Verification items for the finished model (mm, model axes). Face numbers are marked on the shaded views. Give positions to 0.01 mm unless a question says otherwise; leave off trailing zeros. Loops run counter-clockwise (first coordinate to the right, second up) from the corner with the lowest first, then second, coordinate; pieces in that order, holes last. Notation, with made-up numbers: (74.5, 47.25) - (133.5, 47.25) arc R11 cw to (133.5, 65.25) - close; hole circle Ø7 at (81, 78). An arc over 180 degrees is marked (long way). Answer in a Markdown table with one row per item.
```python
from build123d import *

# Parameters (mm, degrees)
F0_R     = 40.1475524572
F0_R_2   = 26.11755
F1_DEPTH = 1.524
F2_DEPTH = 6.096


# Not quite as in the source:
# - a fillet or chamfer that OpenCascade refuses, or shapes differently, is made with other operations: its cross-section is extruded or revolved along the edge and cut away or added


with BuildPart() as f1:
    # F0 (on Front) → F1 (new body)
    with BuildSketch(Plane.XZ):
        Circle(F0_R)
        with Locations((0.0001517863, 0)):
            Circle(F0_R_2, mode=Mode.SUBTRACT)
        with Locations((0.0001517863, 0)):
            Circle(F0_R_2)
        with BuildLine():
            ThreePointArc((0.0001517863, 22.3475835458), (14.93341969, 16.1620214495), (21.1189817863, 1.2287535458))
            ThreePointArc((21.1189817863, 1.2287535458), (-14.9331161175, -13.704514358), (0.0001517863, 22.3475835458))
        make_face(mode=Mode.SUBTRACT)
    extrude(amount=F1_DEPTH)

    # F0 (on Front) → F2 (join)
    with BuildSketch(Plane.XZ):
        with Locations((0.0001517863, 0)):
            Circle(F0_R_2)
        with BuildLine():
            ThreePointArc((0.0001517863, 22.3475835458), (14.93341969, 16.1620214495), (21.1189817863, 1.2287535458))
            ThreePointArc((21.1189817863, 1.2287535458), (-14.9331161175, -13.704514358), (0.0001517863, 22.3475835458))
        make_face(mode=Mode.SUBTRACT)
    extrude(amount=F2_DEPTH)

    # F3: fillet of radius 5.08 on 1 edges, made by hand

    # F3_s1 → F3_t2 (revolve)
    with BuildSketch(Plane.XY):
        with BuildLine():
            ThreePointArc((31.1722379668, -1.524), (27.764470369, -2.8365711686), (26.1177017863, -6.096))
            Line((26.1177017863, -6.096), (26.1177017863, -1.524))
            Line((26.1177017863, -1.524), (31.1722379668, -1.524))
        make_face()
    revolve(axis=Axis((0.0001517863, -1.524, 0), (0, 1, 0)))


solid = f1.part
```
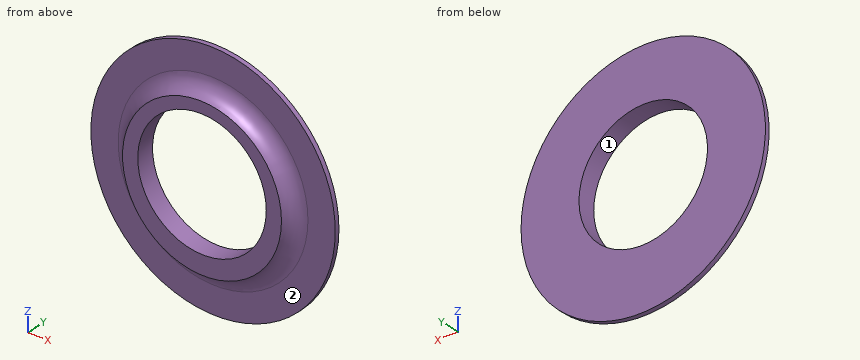
Q1. Go/stop test with flat-tipped pins: P1, Ø3, axis at x = 9.5, z = 26.5, coming from the -Y side; P2, Ø1.5, axis at x = 15, y = -4.5, coming from the -Z side; P3, Ø24, axis at x = 19.5, z = -6, coming from the -Y side; P4, Ø1, axis at x = -27.5, y = -1, coming from the +Z side. Record where each tip stops, or that it passes through.
Completed:
| item | result |
|---|---|
| P1 | y = -4.29 |
| P2 | z = -22.59 |
| P3 | y = -6.1 |
| P4 | z = 29.71 |
Q2. Sectioned sample at C-C (y = -4). Record the cut outline in (x, z).
Completed:
| item | result |
|---|---|
| outline | circle Ø53.62 at (0, 0); hole circle Ø42.24 at (0, 1.23) |
Q3. Sectioned sample at B-B (x = -34). Record the cut outline in (y, z).
Completed:
| item | result |
|---|---|
| outline | (-1.52, -21.35) - (0, -21.35) - (0, 21.35) - (-1.52, 21.35) - close |
Q4. Draft check along X on the marked faces 1 and 2. Enter one of: +X half, -X half, draft (parallel to the pull), parting line (faces both ways), or undercut.
Completed:
| item | result |
|---|---|
| face 1 | undercut |
| face 2 | draft |
Q5. Sectioned sample at D-D (z = 33). Record the cut outline in (x, y), and give its area (3 significant figures).
Completed:
| item | result |
|---|---|
| outline | (-22.87, -1.52) - (22.87, -1.52) - (22.87, 0) - (-22.87, 0) - close |
| area | 69.7 mm^2 |
Q6. Thickness scan on line 1 (X direction, y = -1.25, z = -30.5); line 2 (Z direction, x = -10.5, y = -2.5); line 3 (Z direction, x = -6.5, y = -5.5). Record the ranges inside material, lowest first.
Completed:
| item | result |
|---|---|
| line 1 | -26.11 to 26.11 |
| line 2 | -26.15 to -17.09, 19.55 to 26.15 |
| line 3 | -25.39 to -18.86, 21.32 to 25.39 |
Q7. Sectioned sample at A-A (z = 0). Record the cut outline in (x, y), and give its area (3 significant figures).
Completed:
| item | result |
|---|---|
| outline | (-40.15, -1.52) - (-31.17, -1.52) arc R5.08 cw to (-26.12, -6.1) - (-21.08, -6.1) - (-21.08, 0) - (-40.15, 0) - close; (21.08, -6.1) - (26.12, -6.1) arc R5.08 cw to (31.17, -1.52) - (40.15, -1.52) - (40.15, 0) - (21.08, 0) - close |
| area | 115 mm^2 |
